The listing builds one solid part. Answer for the finished solid, in the listing's coordinates (mm). Face numbers are marked on the shaded views. A direction names the side the tool comes from. Coordinates: 2 decimals unless noted, no trailing zeros. Loops run counter-clockwise (first coordinate to the right, second up) from the corner with the lowest first, then second, coordinate; pieces in that order, holes last. Notation, with made-up numbers: M -19,7 L -5,7 A31 cw -5,44 Z; hole C 43.25,6.5 d8. An arc over 180 degrees is marked long. Return JSON: item names as keys, results as strings. Group by question number.
1. Section A-A (y = 0) is taken. Write down the section's boundary in (x, z), then the cut area to 3 significant figures.
2. Section B-B (x = 8.5) is taken. Write down the section's boundary in (y, z).
3. Straight lines are drawn through the part: L1, parallel to X at y = -0.75, z = -1.25; L2, parallel to X at y = -1.75, z = -1.25; L3, parallel to Y at x = 26, z = 1. For each, find the intervals that lie inside material, in ascending order. Write a range as from..to.
4. Given P1, Ø1.5, axis at x = 49.5, y = -1.5, coming from the -Z side; P2, Ø2, axis at y = 1, z = -3, coming from the -X side; P3, Ø1, axis at y = -0.5, z = -0.5, coming from the -X side; P4, Ø0.5, axis at x = 0.5, y = -0.5, coming from the -Z side, each flat-ended and moving along its own axis, determine where each tip first touches the part or whether it passes through.
5. Which of the six approach directions +Z, -Z, +X, -X, +Y, -Y give full straight-line access (tool end or side, diameter ignored) to the marked faces 1 and 2?
```python
from build123d import *

# Parameters (mm, degrees)
CHAMFER1_SIZE      = 0.3
CUT_EXTRUDE1_DEPTH = 1
CHAMFER2_SIZE      = 0.5


with BuildPart() as part:
    # Sketch1 → Revolve1 (revolve)
    with BuildSketch(Plane.XY):
        Polygon((0, 0), (66, 0), (66, 2), (4, 2), (4, 3.5), (0, 3.5), align=None)
    revolve(axis=Axis((0, 0, 0), (1, 0, 0)))

    # Chamfer1
    chamfer1_edges = [part.edges().sort_by_distance(p)[0] for p in [
        (66, -2, 0),
    ]]
    chamfer(chamfer1_edges, length=CHAMFER1_SIZE)

    # Sketch2 → Cut-Extrude1 (cut)
    with BuildSketch(Plane.ZY):
        Polygon((0, 2), (-1.732050808, 1), (-1.732050808, -1), (0, -2), (1.732050808, -1), (1.732050808, 1), align=None)
    extrude(amount=-CUT_EXTRUDE1_DEPTH, mode=Mode.SUBTRACT)

    # Chamfer2
    chamfer2_edges = [part.edges().sort_by_distance(p)[0] for p in [
        (0, -3.5, 0),
    ]]
    chamfer(chamfer2_edges, length=CHAMFER2_SIZE)


solid = part.part
```
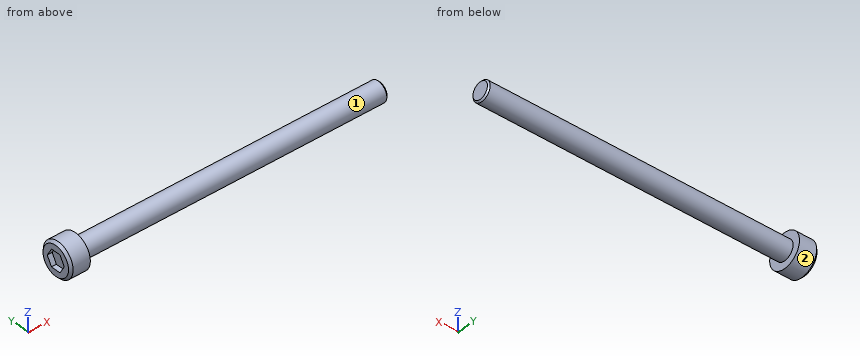
Worked out:
{
 "1": {"outline": "M 0,-3 L 0.5,-3.5 L 4,-3.5 L 4,-2 L 65.7,-2 L 66,-1.7 L 66,1.7 L 65.7,2 L 4,2 L 4,3.5 L 0.5,3.5 L 0,3 L 0,1.73 L 1,1.73 L 1,-1.73 L 0,-1.73 Z", "area": "272 mm^2"},
 "2": {"outline": "C 0,0 d4"},
 "3": {"L1": "1..66", "L2": "0..4", "L3": "-1.73..1.73"},
 "4": {"P1": "z = -1.85", "P2": "x = 0", "P3": "x = 1", "P4": "z = -3.49"},
 "5": {"face 1": "+X", "face 2": "+X, -X"}
}
